Check sheet for the modelled part. Datum: model origin and axes. Units: mm. Face numbers are marked on the shaded views. A direction names the side the tool comes from. Round coordinates to 2 decimals unless told otherwise and drop trailing zeros. Write each loop counter-clockwise with the first axis right and the second up, starting at its lowest first coordinate (ties: lowest second). Pieces come first, ordered by that corner, then holes. Notation, with made-up numbers: (-29.75, 84.25) - (24.25, 84.25) arc R23 cw to (24.25, 105.25) - close; hole circle Ø7 at (87, 6). An arc over 180 degrees is marked (long way). Answer as a JSON object with one key per item and string values. Group by question number.
Item 1: Thickness scan on line 1 (Y direction, x = 1, z = -36); line 2 (Z direction, x = 3, y = 36); line 3 (X direction, y = 35, z = -27.5). Record the ranges inside material, lowest first.
Item 2: Sectioned sample at A-A on x = 30.5. Record the boundary of the cut face in (y, z).
Item 3: Sectioned sample at D-D on x = 15. Record the boundary of the cut face in (y, z), plus the area to 3 significant figures.
Item 4: Set-up check for the marked faces 1, 2 and 3: record each of +Z, -Z, +X, -X, +Y, -Y from which the full face is reachable in a straight line by a thin tool's end or side.
Item 5: Gauge pin test, flat ends, axial feed: P1, Ø3.5, axis at y = 37.5, z = -5, coming from the -X side; P2, Ø16, axis at x = 23.5, z = -19, coming from the +Y side; P3, Ø7.5, axis at x = 33.5, y = 47, coming from the +Z side; P4, Ø3, axis at x = 19, z = -13.5, coming from the +Y side. Record the tip position at first contact, or that the pin passes through.
Item 6: Sectioned sample at B-B on y = 21.15. Record the boundary of the cut face in (x, z).
Item 7: Sectioned sample at C-C on z = -8. Record the boundary of the cut face in (x, y), plus the area to 3 significant figures.
```python
from build123d import *

# Parameters (mm, degrees)
EXTRUDE_2_DEPTH          = 38
SKETCH_2_R               = 11
EXTRUDE_3_DEPTH          = 2
FILLET_1_R               = 1
SKETCH_3_R               = 2.5
EXTRUDE_4_DEPTH          = 20
SKETCH_4_R               = 1.5
CUT_EXTRUDE_1_DEPTH      = 4.5
PATTERN_CIRCULAR_1_COUNT = 4
EXTRUDE_5_DEPTH          = 7


with BuildPart() as part:
    # 草图1 → 凸台-拉伸2 (new body)
    with BuildSketch(Plane(origin=(0, 0, 0), x_dir=(0, 0, -1), z_dir=(1, 0, 0))):
        with BuildLine():
            Line((0.878679656, 39.178679656), (3.121320344, 41.421320344))
            ThreePointArc((3.121320344, 41.421320344), (4.09459039, 42.071638598), (5.242640687, 42.3))
            Line((5.242640687, 42.3), (37.057359313, 42.3))
            ThreePointArc((37.057359313, 42.3), (38.20540961, 42.071638598), (39.178679656, 41.421320344))
            Line((39.178679656, 41.421320344), (41.421320344, 39.178679656))
            ThreePointArc((41.421320344, 39.178679656), (42.071638598, 38.20540961), (42.3, 37.057359313))
            Line((42.3, 37.057359313), (42.3, 5.242640687))
            ThreePointArc((42.3, 5.242640687), (42.071638598, 4.09459039), (41.421320344, 3.121320344))
            Line((41.421320344, 3.121320344), (39.178679656, 0.878679656))
            ThreePointArc((39.178679656, 0.878679656), (38.20540961, 0.228361402), (37.057359313, 0))
            Line((37.057359313, 0), (5.242640687, 0))
            ThreePointArc((5.242640687, 0), (4.09459039, 0.228361402), (3.121320344, 0.878679656))
            Line((3.121320344, 0.878679656), (0.878679656, 3.121320344))
            ThreePointArc((0.878679656, 3.121320344), (0.228361402, 4.09459039), (0, 5.242640687))
            Line((0, 5.242640687), (0, 37.057359313))
            ThreePointArc((0, 37.057359313), (0.228361402, 38.20540961), (0.878679656, 39.178679656))
        make_face()
    extrude(amount=EXTRUDE_2_DEPTH)

    # 草图2 → 凸台-拉伸3 (add)
    with BuildSketch(Plane.ZY):
        with Locations((-21.15, 21.15)):
            Circle(SKETCH_2_R)
    extrude(amount=EXTRUDE_3_DEPTH)

    # 圆角1
    fillet_1_edges = [part.edges().sort_by_distance(p)[0] for p in [
        (-2, 21.15, -32.15),
    ]]
    fillet(fillet_1_edges, radius=FILLET_1_R)

    # 草图3 → 凸台-拉伸4 (add)
    with BuildSketch(Plane.ZY.offset(2)):
        with Locations((-21.15, 21.15)):
            Circle(SKETCH_3_R)
    extrude(amount=EXTRUDE_4_DEPTH)

    # 草图4 → 切除-拉伸1 (cut)
    with BuildSketch(Plane.ZY):
        with Locations((-36.65, 36.65)):
            Circle(SKETCH_4_R)
    cut_extrude_1 = extrude(amount=-CUT_EXTRUDE_1_DEPTH, mode=Mode.SUBTRACT)

    # 阵列(圆周)1: 切除-拉伸1 ×4 about axis
    pattern_circular_1_axis = Axis((0, 21.15, -21.15), (1, 0, 0))
    for i in range(1, PATTERN_CIRCULAR_1_COUNT):
        add(cut_extrude_1.rotate(pattern_circular_1_axis, i * 360 / PATTERN_CIRCULAR_1_COUNT), mode=Mode.SUBTRACT)

    # 草图6 → 凸台-拉伸5 (add)
    with BuildSketch(Plane(origin=(0, 42.3, 0), x_dir=(1, 0, 0), z_dir=(0, 1, 0))):
        Polygon((28.4, 29.967521896), (38, 29.967521896), (38, 13.967521896), (27.87263434, 13.967521896), align=None)
    extrude(amount=EXTRUDE_5_DEPTH)


solid = part.part
```
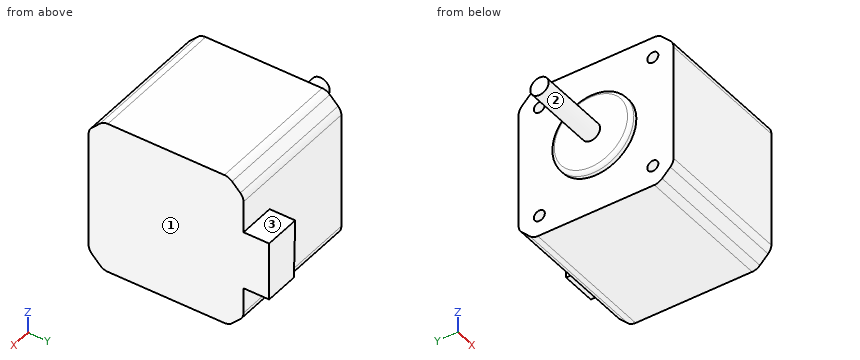
Completed:
{
 "1": {"line 1": "0 to 4.3, 7 to 35.3, 38 to 42.3", "line 2": "-42.3 to -38, -35.3 to -7, -4.3 to 0", "line 3": "0 to 38"},
 "2": {"outline": "(0, -37.06) arc R3 ccw to (0.88, -39.18) - (3.12, -41.42) arc R3 ccw to (5.24, -42.3) - (37.06, -42.3) arc R3 ccw to (39.18, -41.42) - (41.42, -39.18) arc R3 ccw to (42.3, -37.06) - (42.3, -29.97) - (49.3, -29.97) - (49.3, -13.97) - (42.3, -13.97) - (42.3, -5.24) arc R3 ccw to (41.42, -3.12) - (39.18, -0.88) arc R3 ccw to (37.06, 0) - (5.24, 0) arc R3 ccw to (3.12, -0.88) - (0.88, -3.12) arc R3 ccw to (0, -5.24) - close"},
 "3": {"outline": "(0, -37.06) arc R3 ccw to (0.88, -39.18) - (3.12, -41.42) arc R3 ccw to (5.24, -42.3) - (37.06, -42.3) arc R3 ccw to (39.18, -41.42) - (41.42, -39.18) arc R3 ccw to (42.3, -37.06) - (42.3, -5.24) arc R3 ccw to (41.42, -3.12) - (39.18, -0.88) arc R3 ccw to (37.06, 0) - (5.24, 0) arc R3 ccw to (3.12, -0.88) - (0.88, -3.12) arc R3 ccw to (0, -5.24) - close", "area": "1,760 mm²"},
 "4": {"face 1": "+Z, -Z, +X, +Y, -Y", "face 2": "-X", "face 3": "+Z, +X, -X, +Y"},
 "5": {"P1": "x = 0", "P2": "y = 49.3", "P3": "z = -13.97", "P4": "y = 42.3"},
 "6": {"outline": "(-22, -23.65) - (-2, -23.65) - (-2, -31.15) arc R1 ccw to (-1, -32.15) - (0, -32.15) - (0, -42.3) - (38, -42.3) - (38, 0) - (0, 0) - (0, -10.15) - (-1, -10.15) arc R1 ccw to (-2, -11.15) - (-2, -18.65) - (-22, -18.65) - close"},
 "7": {"outline": "(0, 0) - (38, 0) - (38, 42.3) - (0, 42.3) - close", "area": "1,610 mm²"}
}
